```python
from build123d import *

# Parameters (mm, degrees)
F0_W     = 75
F0_H     = 60
F1_DEPTH = 40
F2_W     = 25
F2_H     = 35
F2_W_2   = 24.9936
F2_H_2   = 25
F3_DEPTH = 40.001


with BuildPart() as f1:
    # F0 (on Front) → F1 (new body)
    with BuildSketch(Plane.XZ):
        with Locations((5.865399, -0.198499)):
            Rectangle(F0_W, F0_H)
    extrude(amount=F1_DEPTH)

    # F2 (on Front) → F3 (cut, through all)
    with BuildSketch(Plane.XZ):
        with Locations((-19.235718, 12.4838)):
            Rectangle(F2_W, F2_H)
        with Locations((30.985761, 17.584927)):
            Rectangle(F2_W_2, F2_H_2)
    extrude(amount=F3_DEPTH, mode=Mode.SUBTRACT)


solid = f1.part
```
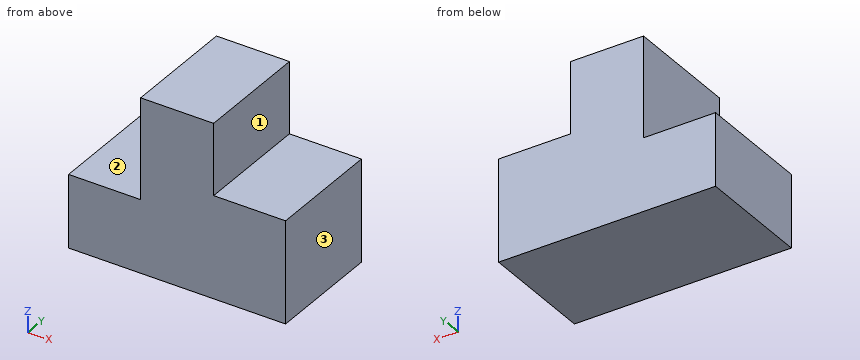
CAD build for the part. Positions are in the model's coordinates, mm. Face numbers are marked on the shaded views. A direction names the side the tool comes from. Round coordinates to 2 decimals unless told otherwise and drop trailing zeros. Write each loop counter-clockwise with the first axis right and the second up, starting at its lowest first coordinate (ties: lowest second). Pieces come first, ordered by that corner, then holes. Notation, with made-up numbers: (40, 16.25) - (81, 16.25) arc R10 cw to (81, 24.25) - close; hole circle Ø1 at (7.5, 44). An arc over 180 degrees is marked (long way). Return JSON: item names as keys, results as strings. Group by question number.
Item 1: 3-axis set-ups, long thin cutter, end or side, ignore diameter. For the marked faces 1, 2 and 3: which of +Z, -Z, +X, -X, +Y, -Y reach the whole face in a straight line?
Item 2: Band-saw the part on B-B on z = 17. List the corners of the cut face in (x, y).
Item 3: Probe probe 1 along Z at (x, y) = (33.5, -10.5); probe 2 along X at (y, z) = (-38, 17.5); probe 3 along Z at (x, y) = (-21, -33). List the from-to ranges inside material, lowest first.
Item 4: Flat gauge pins, fed straight in: pin 1 Ø10.5 at (y, z) = (-13, 12) entering from -X; pin 2 Ø12.5 at (x, y) = (-18.5, -16.5) entering from +Z; pin 3 Ø12 at (y, z) = (-11.5, 15) entering from +X. Where does each tip first touch, or does it go through?
Item 5: Band-saw the part on A-A on y = -17.5. List the corners of the cut face in (x, z).
Item 6: Band-saw the part on C-C on x = 35. List the corners of the cut face in (y, z).
Resolved:
{
 "1": {"face 1": "+Z, +X, +Y, -Y", "face 2": "+Z, -X, +Y, -Y", "face 3": "+Z, -Z, +X, +Y, -Y"},
 "2": {"outline": "(-6.74, -40) - (18.49, -40) - (18.49, 0) - (-6.74, 0) - close"},
 "3": {"probe 1": "z = -30.2 to 5.08", "probe 2": "x = -6.74 to 18.49", "probe 3": "z = -30.2 to -5.02"},
 "4": {"pin 1": "stops at x = -6.74", "pin 2": "stops at z = -5.02", "pin 3": "stops at x = 18.49"},
 "5": {"outline": "(-31.63, -30.2) - (43.37, -30.2) - (43.37, 5.08) - (18.49, 5.08) - (18.49, 29.8) - (-6.74, 29.8) - (-6.74, -5.02) - (-31.63, -5.02) - close"},
 "6": {"outline": "(-40, -30.2) - (0, -30.2) - (0, 5.08) - (-40, 5.08) - close"}
}
